Geometry: final body of the model. Coordinates: model frame, mm. Give positions to 0.01 mm unless a question says otherwise; leave off trailing zeros. Write each loop counter-clockwise with the first axis right and the second up, starting at its lowest first coordinate (ties: lowest second). Pieces come first, ordered by that corner, then holes.
from build123d import *

# Parameters (mm, degrees)
SM_BASE_FLANGE_1_OUTLINE_R = 2.1
SM_BASE_FLANGE_1_DEPTH     = 1.5
CUT_EXTRUDE_2_DEPTH        = 1.5
FILLET_1_R                 = 5
SKETCH_8_R                 = 2.1
CUT_EXTRUDE_5_DEPTH        = 1.5


# Read off the part's stored shape, not the designer's step: 基体-法兰1
with BuildPart() as part:
    # 基体-法兰1 outline → 基体-法兰1 (new body)
    with BuildSketch(Plane.XY):
        with BuildLine():
            ThreePointArc((-20, -148.660687473), (83.338400401, -124.718527167), (145, -38.405728739))
            Line((145, -38.405728739), (145, 38.405728739))
            ThreePointArc((145, 38.405728739), (0, 150), (-145, 38.405728739))
            Line((-145, 38.405728739), (-145, -38.405728739))
            ThreePointArc((-145, -38.405728739), (-102.969737504, -109.074438611), (-30, -146.969384567))
            Line((-30, -146.969384567), (-30, -132.817748132))
            ThreePointArc((-30, -132.817748132), (-25, -127.817748132), (-20, -132.817748132))
            Line((-20, -132.817748132), (-20, -148.660687473))
        make_face()
        with Locations((-36.5, -110)):
            Circle(SM_BASE_FLANGE_1_OUTLINE_R, mode=Mode.SUBTRACT)
        with Locations((-36.5, -70)):
            Circle(SM_BASE_FLANGE_1_OUTLINE_R, mode=Mode.SUBTRACT)
        with Locations((-5, -24.121330526)):
            Circle(SM_BASE_FLANGE_1_OUTLINE_R, mode=Mode.SUBTRACT)
        with BuildLine():
            Line((-14.5, 10), (-14.5, -10))
            ThreePointArc((-14.5, -10), (-16.5, -12), (-18.5, -10))
            Line((-18.5, -10), (-18.5, 10))
            ThreePointArc((-18.5, 10), (-16.5, 12), (-14.5, 10))
        make_face(mode=Mode.SUBTRACT)
        with Locations((36.5, -110)):
            Circle(SM_BASE_FLANGE_1_OUTLINE_R, mode=Mode.SUBTRACT)
        with Locations((36.5, -70)):
            Circle(SM_BASE_FLANGE_1_OUTLINE_R, mode=Mode.SUBTRACT)
        with Locations((5, -24.132256214)):
            Circle(SM_BASE_FLANGE_1_OUTLINE_R, mode=Mode.SUBTRACT)
        Polygon((-10.25, 20.500012235), (10.250024471, 20.522409895), (10.25, -20.522409895), (-10.25, -20.500012235), align=None, mode=Mode.SUBTRACT)
        with BuildLine():
            Line((14.5, -10), (14.5, 10))
            ThreePointArc((14.5, 10), (16.5, 12), (18.5, 10))
            Line((18.5, 10), (18.5, -10))
            ThreePointArc((18.5, -10), (16.5, -12), (14.5, -10))
        make_face(mode=Mode.SUBTRACT)
        with Locations((-5, 24.378698421)):
            Circle(SM_BASE_FLANGE_1_OUTLINE_R, mode=Mode.SUBTRACT)
        with Locations((-5, 86.272395421)):
            Circle(SM_BASE_FLANGE_1_OUTLINE_R, mode=Mode.SUBTRACT)
        with BuildLine():
            Line((-14.5, 120.522409895), (-14.5, 100.522409895))
            ThreePointArc((-14.5, 100.522409895), (-16.5, 98.522409895), (-18.5, 100.522409895))
            Line((-18.5, 100.522409895), (-18.5, 120.522409895))
            ThreePointArc((-18.5, 120.522409895), (-16.5, 122.522409895), (-14.5, 120.522409895))
        make_face(mode=Mode.SUBTRACT)
        with Locations((-5, 134.772424369)):
            Circle(SM_BASE_FLANGE_1_OUTLINE_R, mode=Mode.SUBTRACT)
        with Locations((5, 24.367772734)):
            Circle(SM_BASE_FLANGE_1_OUTLINE_R, mode=Mode.SUBTRACT)
        with Locations((5, 86.261469734)):
            Circle(SM_BASE_FLANGE_1_OUTLINE_R, mode=Mode.SUBTRACT)
        Polygon((-10.25, 90.022397659), (-10.25, 131.02242213), (10.250024471, 131.04481979), (10.25, 90), align=None, mode=Mode.SUBTRACT)
        with BuildLine():
            Line((14.5, 100.522409895), (14.5, 120.522409895))
            ThreePointArc((14.5, 120.522409895), (16.5, 122.522409895), (18.5, 120.522409895))
            Line((18.5, 120.522409895), (18.5, 100.522409895))
            ThreePointArc((18.5, 100.522409895), (16.5, 98.522409895), (14.5, 100.522409895))
        make_face(mode=Mode.SUBTRACT)
        with Locations((5, 134.761498681)):
            Circle(SM_BASE_FLANGE_1_OUTLINE_R, mode=Mode.SUBTRACT)
    extrude(amount=SM_BASE_FLANGE_1_DEPTH)

    # 草图3 → 切除-拉伸2 (cut)
    with BuildSketch(Plane(origin=(0, 0, 0), x_dir=(-1, 0, 0), z_dir=(0, 0, -1))):
        with BuildLine():
            Line((-93.6, -85.709487412), (-93.6, -95.709487412))
            ThreePointArc((-93.6, -95.709487412), (-91, -98.309487412), (-88.4, -95.709487412))
            Line((-88.4, -95.709487412), (-88.4, -85.709487412))
            ThreePointArc((-88.4, -85.709487412), (-91, -83.109487412), (-93.6, -85.709487412))
        make_face()
    extrude(amount=-CUT_EXTRUDE_2_DEPTH, mode=Mode.SUBTRACT)

    # 圆角1
    fillet_1_edges = [part.edges().sort_by_distance(p)[0] for p in [
        (-20, -148.660687473, 0.75),
        (-30, -146.969384567, 0.75),
    ]]
    fillet(fillet_1_edges, radius=FILLET_1_R)

    # 草图8 → 切除-拉伸5 (cut)
    with BuildSketch(Plane.XY.offset(1.5)):
        with Locations(Location((112.770480318, -78.675798494, 0), (0, 0, 180))):
            Circle(SKETCH_8_R)
        with Locations((137, 11.75)):
            Circle(SKETCH_8_R)
        with Locations(Location((137, -11.75, 0), (0, 0, 180))):
            Circle(SKETCH_8_R)
        with Locations((124.520480318, -58.324201506)):
            Circle(SKETCH_8_R)
        with Locations(Location((58.324201506, -124.520480318, 0), (0, 0, 180))):
            Circle(SKETCH_8_R)
        with Locations((78.675798494, -112.770480318)):
            Circle(SKETCH_8_R)
        with Locations(Location((-11.75, -137, 0), (0, 0, 180))):
            Circle(SKETCH_8_R)
        with Locations((11.75, -137)):
            Circle(SKETCH_8_R)
        with Locations(Location((-78.675798494, -112.770480318, 0), (0, 0, 180))):
            Circle(SKETCH_8_R)
        with Locations((-58.324201506, -124.520480318)):
            Circle(SKETCH_8_R)
        with Locations(Location((-124.520480318, -58.324201506, 0), (0, 0, 180))):
            Circle(SKETCH_8_R)
        with Locations((-112.770480318, -78.675798494)):
            Circle(SKETCH_8_R)
        with Locations(Location((-137, 11.75, 0), (0, 0, 180))):
            Circle(SKETCH_8_R)
        with Locations((-137, -11.75)):
            Circle(SKETCH_8_R)
        with Locations(Location((-112.770480318, 78.675798494, 0), (0, 0, 180))):
            Circle(SKETCH_8_R)
        with Locations((-124.520480318, 58.324201506)):
            Circle(SKETCH_8_R)
        with Locations(Location((-58.324201506, 124.520480318, 0), (0, 0, 180))):
            Circle(SKETCH_8_R)
        with Locations((-78.675798494, 112.770480318)):
            Circle(SKETCH_8_R)
        with Locations(Location((11.75, 137, 0), (0, 0, 180))):
            Circle(SKETCH_8_R)
        with Locations((-11.75, 137)):
            Circle(SKETCH_8_R)
        with Locations(Location((78.675798494, 112.770480318, 0), (0, 0, 180))):
            Circle(SKETCH_8_R)
        with Locations((58.324201506, 124.520480318)):
            Circle(SKETCH_8_R)
        with Locations(Location((124.520480318, 58.324201506, 0), (0, 0, 180))):
            Circle(SKETCH_8_R)
        with Locations((112.770480318, 78.675798494)):
            Circle(SKETCH_8_R)
    extrude(amount=-CUT_EXTRUDE_5_DEPTH, mode=Mode.SUBTRACT)


solid = part.part
Q1. Ray query, line 1 along X through (y, z) = (5, 0.5); line 2 along Y through (x, z) = (-114.5, 0.2); line 3 along X through (y, z) = (87, 0.7). Return the intervals inside material, ascending.
Filled sheet:
line 1: x = -145 to -18.5, -14.5 to -10.25, 10.25 to 14.5, 18.5 to 145
line 2: y = -96.9 to -79.87, -77.48 to 77.48, 79.87 to 96.9
line 3: x = -122.19 to -6.97, -3.03 to 3.03, 6.97 to 122.19
Q2. Section C-C on x = -25. Output: boundary loops of the cut face in (y, z), plus the area to 3 significant figures.
Filled sheet:
outline: (-127.82, 0) - (147.9, 0) - (147.9, 1.5) - (-127.82, 1.5) - close
area: 414 mm2
Q3. Pin query (flat end, axial travel): P1, Ø4, axis at x = -58.32, y = -124.52, coming from the -Z side. Return the tip coordinate at first contact, or that it passes through.
Filled sheet:
P1: passes through
Q4. Section B-B on z = 0.75. Count the separate pieces of the cut face and the enclosed holes in it, plus the area to 3 significant figures.
Filled sheet:
separate pieces: 1
enclosed holes: 43
area: 67,300 mm2
Q5. Section A-A on y = 1. Output: boundary loops of the cut face in (x, z).
Filled sheet:
outline: (-145, 0) - (-18.5, 0) - (-18.5, 1.5) - (-145, 1.5) - close; (-14.5, 0) - (-10.25, 0) - (-10.25, 1.5) - (-14.5, 1.5) - close; (10.25, 0) - (14.5, 0) - (14.5, 1.5) - (10.25, 1.5) - close; (18.5, 0) - (145, 0) - (145, 1.5) - (18.5, 1.5) - close
